Check sheet for the modelled part. Datum: model origin and axes. Units: mm. A direction names the side the tool comes from. Coordinates: 2 decimals unless noted, no trailing zeros. Loops run counter-clockwise (first coordinate to the right, second up) from the corner with the lowest first, then second, coordinate; pieces in that order, holes last. Notation, with made-up numbers: (-39.75, 1) - (-21.75, 1) arc R28 cw to (-21.75, 26) - close; hole circle Ø11 at (3.25, -4). An arc over 180 degrees is marked (long way). Write each question's results on one line, items separated by ' | '. Start each with the question number.
1. Thickness scan on line 1 (Y direction, x = 2.3, z = 0); line 2 (Z direction, x = 2.6, y = 8); line 3 (Z direction, x = 1.9, y = -14.5). Record the ranges inside material, lowest first. Write a range as [from, to].
2. Cross-section at B-B (z = -18.5). Record the cut outline in (x, y).
3. Draft check along Z on faces 1 (the face through (2.54, -8.89, -7.55)), 2 (the face through (2.46, 13.64, -18.74)), 3 (the face through (2.465, 5.662, 3.254)). Enter one of: released by +Z, released by -Z, zero draft, split by the parting line, or undercut.
4. Cross-section at C-C (y = 0). Record the cut outline in (x, z), and give its area (3 significant figures).
5. Tool access check on faces 4 (the face through (0, -18, -6)), 5 (the face through (2.535, -1.341, -3.233)), 6 (the face through (2, -40, 5)), 7 (the face through (2, -45, 5.47)), 8 (the face through (2, -25, -6.53)). Record the directions out of +Z, -Z, +X, -X, +Y, -Y that give a thin tool (end or side, any length) a straight path to the whole face; none if there is none.
6. Gauge pin test, flat ends, axial feed: P1, Ø2.5, axis at x = 3, y = -47.5, coming from the +Z side; P2, Ø2, axis at y = -20, z = 6, coming from the +X side; P3, Ø0.5, axis at x = 3.5, z = 4.5, coming from the +Y side; P4, Ø1.5, axis at x = 3.5, z = -1, coming from the -Y side. Record the tip position at first contact, or that the pin passes through.
7. Cross-section at D-D (y = -33). Record the cut outline in (x, z), and give its area (4 significant figures).
8. Cross-section at A-A (z = -1.5). Record the cut outline in (x, y).
```python
from build123d import *

# Parameters (mm, degrees)
CUT_EXTRUDE2_START     = -5
CUT_EXTRUDE2_OUTLINE_R = 3
CUT_EXTRUDE2_DEPTH     = 5
BOSS_EXTRUDE1_START    = -5
BOSS_EXTRUDE1_DEPTH    = 5
BOSS_EXTRUDE2_START    = -5
SKETCH3_R              = 1.5
BOSS_EXTRUDE2_DEPTH    = 5
FILLET1_R              = 2
FILLET2_R              = 5
SKETCH4_R              = 3.5
CUT_EXTRUDE3_DEPTH     = 10
SKETCH5_R              = 1.5
CUT_EXTRUDE4_DEPTH     = 56.120690806


with BuildPart() as part:
    # Cut-Extrude2: read off the stored shape, not the designer's step
    # Cut-Extrude2 outline → Cut-Extrude2 (new body)
    with BuildSketch(Plane(origin=(5, 0, 0), x_dir=(0, 0, -1), z_dir=(1, 0, 0)).offset(CUT_EXTRUDE2_START)):
        with BuildLine():
            ThreePointArc((-6.52418924, 7.07641009), (-6.805902769, 6.805902769), (-7.07641009, 6.52418924))
            ThreePointArc((-7.07641009, 6.52418924), (-6.439370402, 5.019214625), (-5.158353358, 4.004441996))
            ThreePointArc((-5.158353358, 4.004441996), (-5.655362393, 3.265125), (-6.047125175, 2.465044051))
            ThreePointArc((-6.047125175, 2.465044051), (-7.566452573, 3.06705104), (-9.188318666, 2.866256285))
            ThreePointArc((-9.188318666, 2.866256285), (-9.297036078, 2.491133309), (-9.390445525, 2.111908577))
            ThreePointArc((-9.390445525, 2.111908577), (-8.086265665, 1.127082171), (-6.469486047, 0.888771818))
            ThreePointArc((-6.469486047, 0.888771818), (-6.53025, 0), (-6.469486047, -0.888771818))
            ThreePointArc((-6.469486047, -0.888771818), (-8.086265665, -1.127082171), (-9.390445525, -2.111908577))
            ThreePointArc((-9.390445525, -2.111908577), (-9.297036078, -2.491133309), (-9.188318666, -2.866256285))
            ThreePointArc((-9.188318666, -2.866256285), (-7.566452573, -3.06705104), (-6.047125175, -2.465044051))
            ThreePointArc((-6.047125175, -2.465044051), (4.617584058, -4.617584058), (2.465044051, 6.047125175))
            ThreePointArc((2.465044051, 6.047125175), (3.06705104, 7.566452573), (2.866256285, 9.188318666))
            ThreePointArc((2.866256285, 9.188318666), (2.491133309, 9.297036078), (2.111908577, 9.390445525))
            ThreePointArc((2.111908577, 9.390445525), (1.127082171, 8.086265665), (0.888771818, 6.469486047))
            ThreePointArc((0.888771818, 6.469486047), (0, 6.53025), (-0.888771818, 6.469486047))
            ThreePointArc((-0.888771818, 6.469486047), (-1.127082171, 8.086265665), (-2.111908577, 9.390445525))
            ThreePointArc((-2.111908577, 9.390445525), (-2.491133309, 9.297036078), (-2.866256285, 9.188318666))
            ThreePointArc((-2.866256285, 9.188318666), (-3.06705104, 7.566452573), (-2.465044051, 6.047125175))
            ThreePointArc((-2.465044051, 6.047125175), (-3.265125, 5.655362393), (-4.004441996, 5.158353358))
            ThreePointArc((-4.004441996, 5.158353358), (-5.019214625, 6.439370402), (-6.52418924, 7.07641009))
        make_face()
        Circle(CUT_EXTRUDE2_OUTLINE_R, mode=Mode.SUBTRACT)
    extrude(amount=CUT_EXTRUDE2_DEPTH)

    # Sketch2 → Boss-Extrude1 (add)
    with BuildSketch(Plane(origin=(5, 0, 0), x_dir=(0, 0, -1), z_dir=(1, 0, 0)).offset(BOSS_EXTRUDE1_START)):
        with BuildLine():
            Line((-3.71975, -10.353236172), (-3.71975, -40))
            Line((-3.71975, -40), (-5.46975, -40))
            Line((-5.46975, -40), (-5.46975, -50))
            ThreePointArc((-5.46975, -50), (3.015531374, -46.485281374), (6.53025, -38))
            Line((6.53025, -38), (6.53025, 0))
            ThreePointArc((6.53025, 0), (2.085463632, -6.188295929), (-5.198246307, -3.952518235))
            ThreePointArc((-5.198246307, -3.952518235), (-3.771697436, -6.994118204), (-3.71975, -10.353236172))
        make_face()
    extrude(amount=BOSS_EXTRUDE1_DEPTH)

    # Sketch3 → Boss-Extrude2 (add)
    with BuildSketch(Plane(origin=(5, 0, 0), x_dir=(0, 0, -1), z_dir=(1, 0, 0)).offset(BOSS_EXTRUDE2_START)):
        with BuildLine():
            Line((6.53025, 0), (6.53025, -7.78173689))
            ThreePointArc((6.53025, -7.78173689), (18.005815569, -2.228753726), (22.655916213, 9.64141018))
            ThreePointArc((22.655916213, 9.64141018), (18.655916213, 13.64141018), (14.655916213, 9.64141018))
            ThreePointArc((14.655916213, 9.64141018), (12.257472566, 3.739621168), (6.422011938, 1.184030293))
            ThreePointArc((6.422011938, 1.184030293), (6.503134187, 0.594483644), (6.53025, 0))
        make_face()
        with Locations((18.655916213, 9.64141018)):
            Circle(SKETCH3_R, mode=Mode.SUBTRACT)
    extrude(amount=BOSS_EXTRUDE2_DEPTH)

    # Fillet1
    fillet1_edges = [part.edges().sort_by_distance(p)[0] for p in [
        (2.5, 1.184030293, -6.422011938),
    ]]
    fillet(fillet1_edges, radius=FILLET1_R)

    # Fillet2
    fillet2_edges = [part.edges().sort_by_distance(p)[0] for p in [
        (2.5, -7.78173689, -6.53025),
    ]]
    fillet(fillet2_edges, radius=FILLET2_R)

    # Sketch4 → Cut-Extrude3 (cut)
    with BuildSketch(Plane(origin=(5, 0, 0), x_dir=(0, 0, -1), z_dir=(1, 0, 0))):
        Circle(SKETCH4_R)
    extrude(amount=-CUT_EXTRUDE3_DEPTH, mode=Mode.SUBTRACT)

    # Sketch5 → Cut-Extrude4 (cut, through all)
    with BuildSketch(Plane.ZY):
        with Locations((-1.28025, -14.410797367)):
            Circle(SKETCH5_R)
        with Locations((-1.28025, -39.410797367)):
            Circle(SKETCH5_R)
    extrude(amount=-CUT_EXTRUDE4_DEPTH, mode=Mode.SUBTRACT)


solid = part.part
```
Established:
1) line 1: [-48.68, -40.19], [-38.63, -15.19], [-13.63, -3.5], [3.5, 6.53] | line 2: [-22.58, -14.5], [-3.09, -1.09], [1.09, 3.09] | line 3: [-6.53, -2.78], [0.22, 3.72]
2) outline: (0, -1.67) - (5, -1.67) - (5, 8.15) - (0, 8.15) - close; (0, 11.13) - (5, 11.13) - (5, 13.64) - (0, 13.64) - close
3) face 1: released by -Z | face 2: split by the parting line | face 3: undercut
4) outline: (0, -19.76) - (5, -19.76) - (5, -3.5) - (0, -3.5) - close; (0, 3.5) - (5, 3.5) - (5, 6.53) - (0, 6.53) - close | area: 96.4 mm^2
5) face 4: +Z, -Z, -X, +Y, -Y | face 5: +X, -X | face 6: +Z, +X, -X | face 7: +Z, +X, -X, -Y | face 8: -Z, +X, -X, -Y
6) P1: z = 5.47 | P2: through | P3: y = 6.21 | P4: y = -48.55
7) outline: (0, -6.53) - (5, -6.53) - (5, 3.72) - (0, 3.72) - close | area: 51.25 mm^2
8) outline: (0, -47.77) - (5, -47.77) - (5, -40.89) - (0, -40.89) - close; (0, -37.93) - (5, -37.93) - (5, -15.89) - (0, -15.89) - close; (0, -12.93) - (5, -12.93) - (5, -3.16) - (0, -3.16) - close; (0, 3.16) - (5, 3.16) - (5, 8.75) - (0, 8.75) - close
